Design review of the part built by this model. Coordinates are the model's own, in mm. A direction names the side the tool comes from. Give positions to 0.01 mm unless a question says otherwise; leave off trailing zeros. Loops run counter-clockwise (first coordinate to the right, second up) from the corner with the lowest first, then second, coordinate; pieces in that order, holes last. Notation, with made-up numbers: M -10.75,62 L 9.25,62 A22 cw 9.25,85 Z; hole C -10,83.25 d2. An arc over 180 degrees is marked long. Use a Markdown table: item, result. Add a question column.
(1) Insertion check: pin 1 Ø5.5 at (x, z) = (61.5, 3) entering from -Y; pin 2 Ø4 at (x, z) = (60.5, 3) entering from +Y; pin 3 Ø3 at (y, z) = (27, 11.5) entering from +X. Each pin has a flat end and moves straight along its axis. Give the tip position at first contact, or say it passes through.
(2) Add section B-B, the plane z = 3. Give the boundary of the cut face in (x, y).
(3) Add section A-A, the plane y = 26. Give the boundary of the cut face in (x, z).
(4) For faces 1 (the face through (-4, 12.5, 2)), 2 (the face through (62, 20, 5)), 3 (the face through (-4, 20, 5)), list the 3-axis set-ups (+Z, -Z, +X, -X, +Y, -Y) from which the entire face can be reached by the end or side of a thin tool; tool diameter is ignored.
(5) For probe 1 along X at (y, z) = (22.5, 13.75); probe 2 along Y at (x, z) = (59, 3.25); probe 3 along Z at (x, y) = (-3, 19), list the stretches that pass through material, from the lowest coordinate up.
(6) Add section C-C, the plane z = 12.75. Give the boundary of the cut face in (x, y).
```python
from build123d import *

# Parameters (mm, degrees)
BOX002_W     = 8
BOX002_H     = 15
BOX002_DEPTH = 5
BOX001_W     = 8
BOX001_H     = 15
BOX001_DEPTH = 5
BOX_W        = 58
BOX_H        = 40
BOX_DEPTH    = 22.5


with BuildPart() as obj1:
    # Box002 → Box002 (new body)
    with BuildSketch(Plane(origin=(-8, 12.5, 0), x_dir=(1, 0, 0), z_dir=(0, 0, 1))):
        with Locations((4, 7.5)):
            Rectangle(BOX002_W, BOX002_H)
    extrude(amount=BOX002_DEPTH)


with BuildPart() as obj2:
    # Box001 → Box001 (new body)
    with BuildSketch(Plane(origin=(58, 12.5, 0), x_dir=(1, 0, 0), z_dir=(0, 0, 1))):
        with Locations((4, 7.5)):
            Rectangle(BOX001_W, BOX001_H)
    extrude(amount=BOX001_DEPTH)


with BuildPart() as fusion:
    # Box → Box (new body)
    with BuildSketch(Plane.XY):
        with Locations((29, 20)):
            Rectangle(BOX_W, BOX_H)
    extrude(amount=BOX_DEPTH)

    # Fusion: union obj1, obj2
    add(obj1.part)
    add(obj2.part)


solid = fusion.part
```
Established:
| question | item | result |
|---|---|---|
| 1 | pin 1 | y = 12.5 |
| 1 | pin 2 | y = 27.5 |
| 1 | pin 3 | x = 58 |
| 2 | outline | M -8,12.5 L 0,12.5 L 0,0 L 58,0 L 58,12.5 L 66,12.5 L 66,27.5 L 58,27.5 L 58,40 L 0,40 L 0,27.5 L -8,27.5 Z |
| 3 | outline | M -8,0 L 66,0 L 66,5 L 58,5 L 58,22.5 L 0,22.5 L 0,5 L -8,5 Z |
| 4 | face 1 | +Z, -Z, -X, -Y |
| 4 | face 2 | +Z, +X, +Y, -Y |
| 4 | face 3 | +Z, -X, +Y, -Y |
| 5 | probe 1 | 0 to 58 |
| 5 | probe 2 | 12.5 to 27.5 |
| 5 | probe 3 | 0 to 5 |
| 6 | outline | M 0,0 L 58,0 L 58,40 L 0,40 Z |
